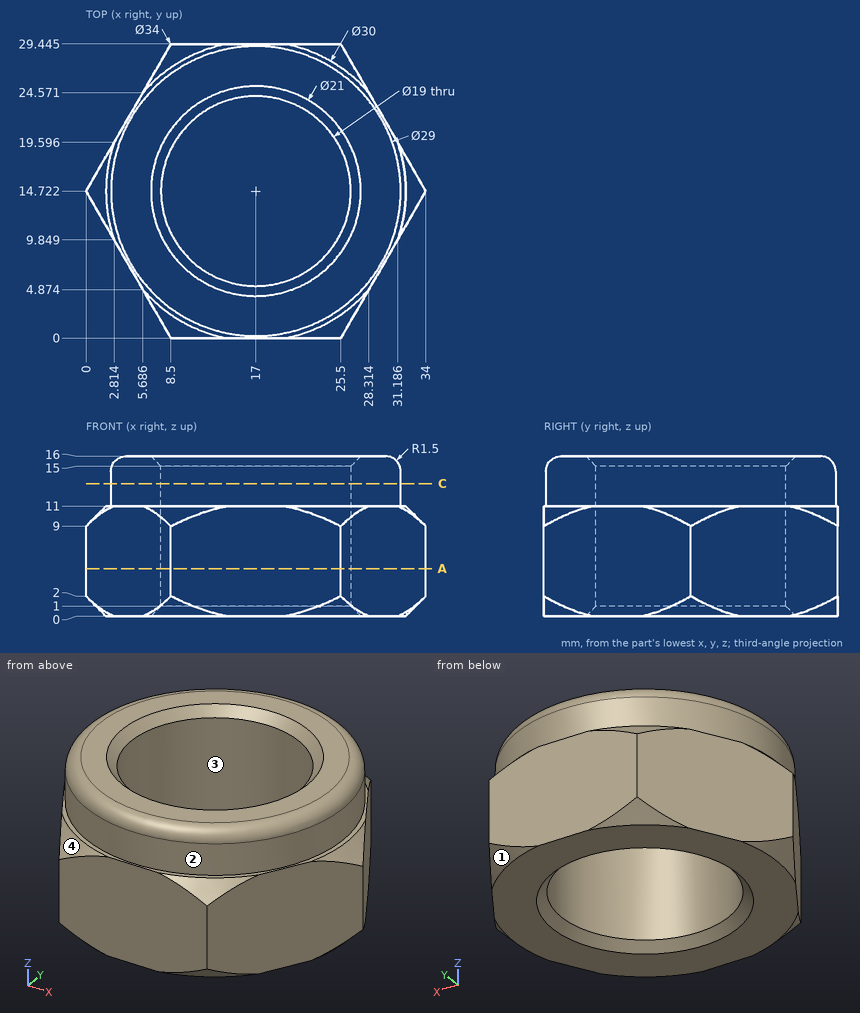
Here's the drawing with two shaded views (mm, measured from the low corner). I have some questions. Coordinates: 2 decimals unless noted, no trailing zeros. Order: outer loops, then holes, each group sorted by start corner. A loop starts at its lowest first (then second) coordinate and runs counter-clockwise, first axis right, second up.
Item 1: If we section it at C-C on z = 13.25: List the corners of the cut face in (x, y) for me, plus the area to 3 significant figures.
Result sheet:
outline: circle Ø29 at (17, 14.72); hole circle Ø19 at (17, 14.72)
area: 377 mm2
Item 2: For P1, Ø12, axis at x = 14, y = 18, coming from the +Z side (1 decimal); P2, Ø1.5, axis at x = 19, z = 11.5, coming from the -Y side; P3, Ø1.5, axis at x = 4.5, z = 6.5, coming from the +Y side (1 decimal); P4, Ø4, axis at y = 26.5, z = 11.5, coming from the +X side, each with a flat end and sliding along its axis, tell me the tip position at first contact or that it passes through.
Result sheet:
P1: stops at z = 15.9
P2: stops at y = 0
P3: stops at y = 23.8
P4: stops at x = 28.32
Item 3: If we mould it in two halves opening along X, with no side actions, what happens to the marked faces 1, 2, 3 and 4? For each: +X half, -X half, draft (parallel to the pull), parting line (faces both ways), or undercut.
Result sheet:
face 1: +X half
face 2: parting line
face 3: undercut
face 4: -X half
Item 4: If we section it at A-A on z = 4.75: List the corners of the cut face in (x, y) for me (1 decimal).
Result sheet:
outline: (0, 14.7) - (8.5, 0) - (25.5, 0) - (34, 14.7) - (25.5, 29.4) - (8.5, 29.4) - close; hole circle Ø19 at (17, 14.7)
Item 5: I need wall thicknesses on line 1 (Y direction, x = 17, z = 8.75) (1 decimal); line 2 (Y direction, x = 17, z = 11.75); line 3 (X direction, y = 8, z = 2.25) (1 decimal). Which ranges of each line are inside material? Lowest first, please.
Result sheet:
line 1: y = 0 to 5.2, 24.2 to 29.4
line 2: y = 0.22 to 5.22, 24.22 to 29.22
line 3: x = 3.9 to 10.3, 23.7 to 30.1
